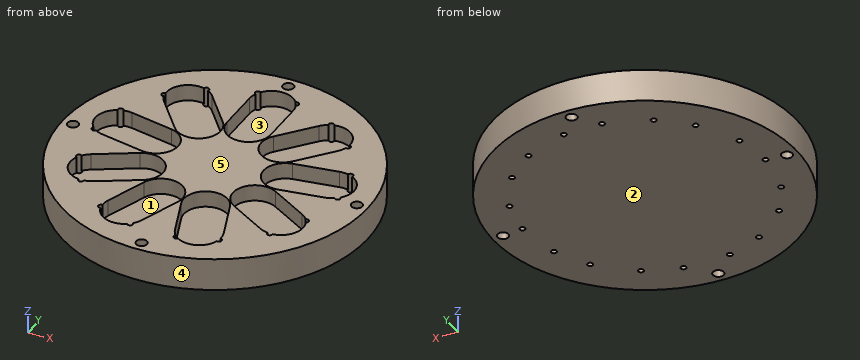
from build123d import *

# Parameters (mm, degrees)
SKETCH_R              = 70
PAD_DEPTH             = 15
POCKET_DEPTH          = 7.5
POLARPATTERN_COUNT    = 9
SKETCH002_R           = 1.25
POCKET001_DEPTH       = 15
POLARPATTERN001_COUNT = 9
SKETCH003_R           = 2.5
POCKET002_DEPTH       = 412.115593
POLARPATTERN002_COUNT = 4


with BuildPart() as part:
    # Sketch (on PolarPattern) → Pad (new body)
    with BuildSketch(Plane.XY):
        Circle(SKETCH_R)
    extrude(amount=PAD_DEPTH)

    # Sketch001 (on Face3 of Pad) → Pocket (cut)
    with BuildSketch(Plane.XY.offset(15)):
        with BuildLine():
            ThreePointArc((10, 50), (0, 60), (-10, 50))
            Line((-10, 50), (-10, 30))
            ThreePointArc((-10, 30), (0, 20), (10, 30))
            Line((10, 50), (10, 30))
        make_face()
    pocket = extrude(amount=-POCKET_DEPTH, mode=Mode.SUBTRACT)

    # PolarPattern: Pocket ×9 about axis
    polarpattern_axis = Axis((0, 0, 15), (0, 0, 1))
    for i in range(1, POLARPATTERN_COUNT):
        add(pocket.rotate(polarpattern_axis, i * 360 / POLARPATTERN_COUNT), mode=Mode.SUBTRACT)

    # Sketch002 (on Face3 of Pad) → Pocket001 (cut)
    with BuildSketch(Plane.XY.offset(15)):
        with Locations((-8.75, 55)):
            Circle(SKETCH002_R)
        with Locations((8.75, 55)):
            Circle(SKETCH002_R)
    pocket001 = extrude(amount=-POCKET001_DEPTH, mode=Mode.SUBTRACT)

    # PolarPattern001: Pocket001 ×9 about axis
    polarpattern001_axis = Axis((0, 0, 15), (0, 0, 1))
    for i in range(1, POLARPATTERN001_COUNT):
        add(pocket001.rotate(polarpattern001_axis, i * 360 / POLARPATTERN001_COUNT), mode=Mode.SUBTRACT)

    # Sketch003 (on Face3 of PolarPattern001) → Pocket002 (cut, through all)
    with BuildSketch(Plane.XY.offset(15)):
        with Locations((0, 65)):
            Circle(SKETCH003_R)
    pocket002 = extrude(amount=-POCKET002_DEPTH, mode=Mode.SUBTRACT)

    # PolarPattern002: Pocket002 ×4 about axis
    polarpattern002_axis = Axis((0, 0, 15), (0, 0, 1))
    for i in range(1, POLARPATTERN002_COUNT):
        add(pocket002.rotate(polarpattern002_axis, i * 360 / POLARPATTERN002_COUNT), mode=Mode.SUBTRACT)


solid = part.part
Read the model definition and answer for the solid it produces. Units are mm, in the model's axes. Face numbers are marked on the shaded views. A direction names the side the tool comes from. Round coordinates to 2 decimals unless told otherwise and drop trailing zeros. Write each loop counter-clockwise with the first axis right and the second up, starting at its lowest first coordinate (ties: lowest second). Pieces come first, ordered by that corner, then holes.
1. Which of the six approach directions +Z, -Z, +X, -X, +Y, -Y give full straight-line access (tool end or side, diameter ignored) to the marked faces 1 and 2?
2. Determine the mould class of the marked faces 3, 4 and 5 for opening direction X: pulls with the +X half, pulls with the -X half, needs draft (parallel to the pull), parting line crosses it, or undercut.
3. The part is cut by section A-A, the plane x = -65. Determine the outline of the cut face in (y, z).
4. The part is cut by section C-C, the plane y = -40. Determine the outline of the cut face in (x, z).
5. The part is cut by section D-D, the plane x = -34. Determine the outline of the cut face in (y, z).
6. Straight lines are drawn through the part: L1, parallel to X at y = 55, z = 7; L2, parallel to X at y = -51.5, z = 11.5; L3, parallel to X at y = -0.5, z = 12.25. For each, find the intervals that lie inside material, in ascending order.
7. Given pin 1 Ø1 at (y, z) = (-36.5, 12.5) entering from +X; pin 2 Ø1.5 at (x, z) = (-6, 8.5) entering from +Y; pin 3 Ø1.5 at (y, z) = (9.5, 8) entering from -X, each flat-ended and moving along its own axis, determine where each tip first touches the part or whether it passes through.
Values:
1. face 1: +Z
1. face 2: -Z, +X, -X, +Y, -Y
2. face 3: undercut
2. face 4: parting line crosses it
2. face 5: needs draft
3. outline: (-25.98, 0) - (-2.5, 0) - (-2.5, 15) - (-25.98, 15) - close; (2.5, 0) - (25.98, 0) - (25.98, 15) - (2.5, 15) - close
4. outline: (-57.45, 0) - (57.45, 0) - (57.45, 15) - (25.2, 15) - (25.2, 7.5) - (3.92, 7.5) - (3.92, 15) - (-3.92, 15) - (-3.92, 7.5) - (-25.2, 7.5) - (-25.2, 15) - (-57.45, 15) - close
5. outline: (-61.19, 0) - (61.19, 0) - (61.19, 15) - (48.13, 15) - (48.13, 7.5) - (24.96, 7.5) - (24.96, 15) - (16.15, 15) - (16.15, 7.5) - (-4.16, 7.5) - (-4.16, 15) - (-8.08, 15) - (-8.08, 7.5) - (-31.18, 7.5) - (-31.18, 15) - (-61.19, 15) - close
6. L1: x = -43.3 to -10, -7.5 to 7.5, 10 to 43.3
6. L2: x = -47.41 to -26.02, -8.18 to 8.18, 26.02 to 47.41
6. L3: x = -70 to -67.45, -62.55 to -53.2, -21.33 to 21.33, 53.2 to 62.55, 67.45 to 70
7. pin 1: stops at x = 60.03
7. pin 2: stops at y = 69.8
7. pin 3: stops at x = -69.45
